Source: CAD feature listing. Evaluate the final solid. Frame: model axes, mm. Face numbers are marked on the shaded views. A direction names the side the tool comes from. Coordinates: 2 decimals unless noted, no trailing zeros. Order: outer loops, then holes, each group sorted by start corner. A loop starts at its lowest first (then second) coordinate and runs counter-clockwise, first axis right, second up.
```python
from build123d import *

# Parameters (mm, degrees)
SKETCH_R     = 11
PAD_DEPTH    = 3
SKETCH001_R  = 5
POCKET_DEPTH = 1
SKETCH002_R  = 5.1
PAD001_DEPTH = 14
CHAMFER_SIZE = 0.9


with BuildPart() as part:
    # Sketch → Pad (new body)
    with BuildSketch(Plane.XY):
        Circle(SKETCH_R)
    extrude(amount=PAD_DEPTH)

    # Sketch001 (on Face3 of Pad) → Pocket (cut)
    with BuildSketch(Plane.XY.offset(3)):
        Circle(SKETCH001_R)
    extrude(amount=-POCKET_DEPTH, mode=Mode.SUBTRACT)

    # Sketch002 (on Face2 of Pocket) → Pad001 (join)
    with BuildSketch(Plane(origin=(0, 0, 0), x_dir=(1, 0, 0), z_dir=(0, 0, -1))):
        Circle(SKETCH002_R)
    extrude(amount=PAD001_DEPTH)

    # Chamfer
    chamfer_edges = [part.edges().sort_by_distance(p)[0] for p in [
        (-5, 0, 3),
    ]]
    chamfer(chamfer_edges, length=CHAMFER_SIZE)


solid = part.part
```
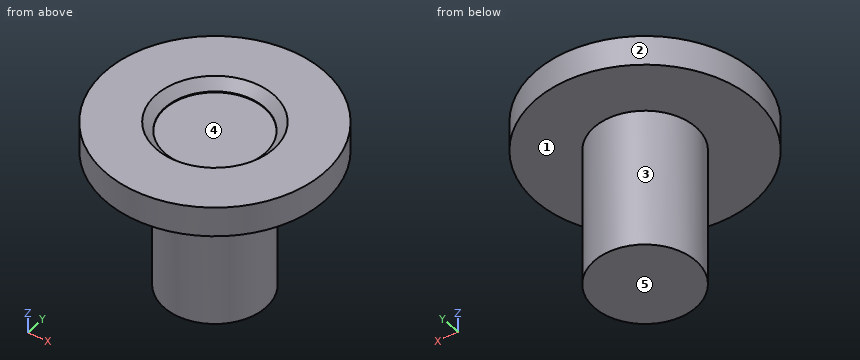
1. Section query A-A on x = 0. Return loops of the section in (y, z), plus the area to 3 significant figures.
Findings:
outline: (-11, 0) - (-5.1, 0) - (-5.1, -14) - (5.1, -14) - (5.1, 0) - (11, 0) - (11, 3) - (5.9, 3) - (5, 2.1) - (5, 2) - (-5, 2) - (-5, 2.1) - (-5.9, 3) - (-11, 3) - close
area: 198 mm2
2. Ray query, line 1 (Y direction, x = 0, z = 2.1); line 2 (Z direction, x = -8.5, y = 6); line 3 (Z direction, x = 0.5, y = -2). Return the intervals inside material, ascending.
Findings:
line 1: y = -11 to -5, 5 to 11
line 2: z = 0 to 3
line 3: z = -14 to 2
3. Section query C-C on z = 0.75. Return loops of the section in (x, y), plus the area to 3 significant figures.
Findings:
outline: circle Ø22 at (0, 0)
area: 380 mm2
4. Section query D-D on z = -5.5. Return loops of the section in (x, y).
Findings:
outline: circle Ø10.2 at (0, 0)
5. Access query for the marked faces 1 and 2. Directions: +Z, -Z, +X, -X, +Y, -Y. A direction counts if a zero-diameter tool reaches every point of the face in a straight line with its end or side. Return the directions, or none.
Findings:
face 1: -Z
face 2: +Z, -Z
6. Pin query (flat end, axial travel): P1, Ø10, axis at y = -3.5, z = -8.5, coming from the -X side; P2, Ø3, axis at x = 7.5, z = -4.5, coming from the -Y side; P3, Ø3, axis at x = 0, y = -2, coming from the +Z side; P4, Ø3, axis at x = 2, z = -2.5, coming from the +Y side. Return the tip coordinate at first contact, or that it passes through.
Findings:
P1: stops at x = -5.1
P2: passes through
P3: stops at z = 2
P4: stops at y = 5.08
7. Draft query along Y for the marked faces 3, 4 and 5. Return one class per face: released by +Y, released by -Y, zero draft, split by the parting line, or undercut.
Findings:
face 3: split by the parting line
face 4: undercut
face 5: zero draft
